Verification items for the finished model (mm, model axes). Face numbers are marked on the shaded views. A direction names the side the tool comes from. Give positions to 0.01 mm unless a question says otherwise; leave off trailing zeros. Write each loop counter-clockwise with the first axis right and the second up, starting at its lowest first coordinate (ties: lowest second). Pieces come first, ordered by that corner, then holes. Notation, with made-up numbers: (11.5, 13.5) - (56.5, 13.5) arc R9 ccw to (56.5, 26.5) - close; hole circle Ø10 at (-4, 39). An arc over 180 degrees is marked (long way). Put each result on its own line as item: value.
from build123d import *

# Parameters (mm, degrees)
SKETCH1_R           = 2
BOSS_EXTRUDE1_DEPTH = 1.6
SKETCH1_3_W         = 8.2
SKETCH1_3_H         = 8.2
SKETCH1_3_W_2       = 6.2
SKETCH1_3_H_2       = 6.2
BOSS_EXTRUDE2_DEPTH = 2
BOSS_EXTRUDE3_START = -0.5
SKETCH1_4_W         = 8.2
SKETCH1_4_H         = 8.2
SKETCH1_4_W_2       = 6.2
SKETCH1_4_H_2       = 6.2
SKETCH1_4_R         = 2
BOSS_EXTRUDE3_DEPTH = 0.5
SKETCH3_W           = 5.8
SKETCH3_H           = 5.8
BOSS_EXTRUDE4_DEPTH = 4.5
CHAMFER1_SIZE       = 0.5
CUT_EXTRUDE1_DEPTH  = 0.2


with BuildPart() as part:
    # Sketch1 → Boss-Extrude1 (new body)
    with BuildSketch(Plane(origin=(0, 0, 0), x_dir=(1, 0, 0), z_dir=(0, 1, 0))):
        with Locations(Location((0, 0, 0), (0, 0, 270))):
            Circle(SKETCH1_R)
    extrude(amount=BOSS_EXTRUDE1_DEPTH)



with BuildPart() as body_2:
    # Sketch1_3 → Boss-Extrude2 (new body)
    with BuildSketch(Plane(origin=(0, 0, 0), x_dir=(1, 0, 0), z_dir=(0, 1, 0))):
        Rectangle(SKETCH1_3_W, SKETCH1_3_H)
        Rectangle(SKETCH1_3_W_2, SKETCH1_3_H_2, mode=Mode.SUBTRACT)
    extrude(amount=BOSS_EXTRUDE2_DEPTH)


with BuildPart() as part_1:
    add(part.part)

    add(body_2.part)  # Boss-Extrude3 merges body 2
    # Sketch1_4 → Boss-Extrude3 (add)
    # profile 1 of 3: a face of its own
    with BuildSketch(Plane(origin=(0, 0, 0), x_dir=(1, 0, 0), z_dir=(0, 1, 0)).offset(BOSS_EXTRUDE3_START)):
        Rectangle(SKETCH1_4_W, SKETCH1_4_H)
        Rectangle(SKETCH1_4_W_2, SKETCH1_4_H_2, mode=Mode.SUBTRACT)
    # profile 2 of 3: a face of its own
    with BuildSketch(Plane(origin=(0, 0, 0), x_dir=(1, 0, 0), z_dir=(0, 1, 0)).offset(BOSS_EXTRUDE3_START)):
        Rectangle(SKETCH1_4_W_2, SKETCH1_4_H_2)
        with Locations(Location((0, 0, 0), (0, 0, 270))):
            Circle(SKETCH1_4_R, mode=Mode.SUBTRACT)
    # profile 3 of 3: a face of its own
    with BuildSketch(Plane(origin=(0, 0, 0), x_dir=(1, 0, 0), z_dir=(0, 1, 0)).offset(BOSS_EXTRUDE3_START)):
        with Locations(Location((0, 0, 0), (0, 0, 270))):
            Circle(SKETCH1_4_R)
    extrude(amount=BOSS_EXTRUDE3_DEPTH)

    # Sketch3 → Boss-Extrude4 (add)
    with BuildSketch(Plane.XZ.offset(0.5)):
        Rectangle(SKETCH3_W, SKETCH3_H)
    extrude(amount=BOSS_EXTRUDE4_DEPTH)

    # Chamfer1
    chamfer1_edges = [part_1.edges().sort_by_distance(p)[0] for p in [
        (2.9, -2.75, -2.9),
        (2.9, -2.75, 2.9),
        (-2.9, -2.75, 2.9),
        (-2.9, -2.75, -2.9),
        (-4.1, 0.75, -4.1),
        (4.1, 0.75, -4.1),
        (4.1, 0.75, 4.1),
        (-4.1, 0.75, 4.1),
    ]]
    chamfer(chamfer1_edges, length=CHAMFER1_SIZE)

    # Sketch4 → Cut-Extrude1 (cut)
    with BuildSketch(Plane.XZ.offset(5)):
        Polygon((0.178918545, 2.162051717), (1.79430316, -1.337948283), (1.452856846, -1.337948283), (0.935428962, -0.216153411), (-0.65120966, -0.216153411), (-1.183361102, -1.337948283), (-1.52620966, -1.337948283), (0.13404675, 2.162051717), align=None)
        Polygon((0.152977039, 1.479860211), (-0.480837064, 0.142820948), (0.769964218, 0.142820948), align=None, mode=Mode.SUBTRACT)
    extrude(amount=-CUT_EXTRUDE1_DEPTH, mode=Mode.SUBTRACT)


solid = part_1.part
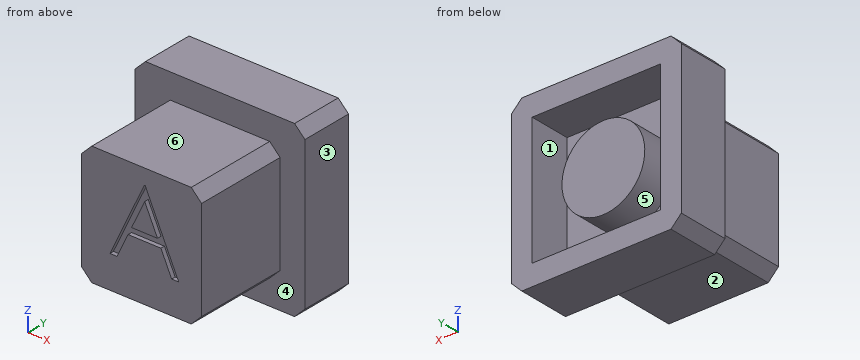
Q1. Scan lines: line 1 along X through (y, z) = (1.5, 0); line 2 along X through (y, z) = (1, -2.25). Record each from-to range of solid material in increasing order.
Answers follow:
line 1: x = -4.1 to -3.1, -2 to 2, 3.1 to 4.1
line 2: x = -4.1 to -3.1, 3.1 to 4.1
Q2. Release check for a two-part mould opening along X. For the marked faces 1, 2 and 3 record: released by +X, released by -X, zero draft, split by the parting line, or undercut.
Answers follow:
face 1: undercut
face 2: zero draft
face 3: released by +X
Q3. Section check B-B, the plane z = -2.75. Record the cut outline in (x, y).
Answers follow:
outline: (-4.1, -0.5) - (-2.55, -0.5) - (-2.55, -5) - (2.55, -5) - (2.55, -0.5) - (4.1, -0.5) - (4.1, 2) - (3.1, 2) - (3.1, 0) - (-3.1, 0) - (-3.1, 2) - (-4.1, 2) - close
Q4. Go/stop test with flat-tipped pins: pin 1 Ø2 at (x, z) = (-0.5, -0.5) entering from +Y; pin 2 Ø4 at (y, z) = (-3, 0.5) entering from +X; pin 3 Ø1.3 at (y, z) = (-2, 0.5) entering from -X. Record where each tip stops, or that it passes through.
Answers follow:
pin 1: stops at y = 1.6
pin 2: stops at x = 2.9
pin 3: stops at x = -2.9
Q5. Set-up check for the marked faces 4, 5 and 6: record each of +Z, -Z, +X, -X, +Y, -Y from which the full face is reachable in a straight line by a thin tool's end or side.
Answers follow:
face 4: -Y
face 5: +Y
face 6: +Z, +X, -X, -Y
Q6. Section check D-D, the plane y = -1.25. Record the cut outline in (x, z), plus the area to 3 significant figures.
Answers follow:
outline: (-2.9, -2.4) - (-2.4, -2.9) - (2.4, -2.9) - (2.9, -2.4) - (2.9, 2.4) - (2.4, 2.9) - (-2.4, 2.9) - (-2.9, 2.4) - close
area: 33.1 mm2
Q7. Section check A-A, the plane y = 0.5. Record the cut outline in (x, z).
Answers follow:
outline: (-4.1, -3.6) - (-3.6, -4.1) - (3.6, -4.1) - (4.1, -3.6) - (4.1, 3.6) - (3.6, 4.1) - (-3.6, 4.1) - (-4.1, 3.6) - close; circle Ø4 at (0, 0); hole (-3.1, -3.1) - (3.1, -3.1) - (3.1, 3.1) - (-3.1, 3.1) - close
Q8. Section check C-C, the plane x = 2.25. Record the cut outline in (y, z), plus the area to 3 significant figures.
Answers follow:
outline: (-5, -2.9) - (-0.5, -2.9) - (-0.5, -4.1) - (2, -4.1) - (2, -3.1) - (0, -3.1) - (0, 3.1) - (2, 3.1) - (2, 4.1) - (-0.5, 4.1) - (-0.5, 2.9) - (-5, 2.9) - close
area: 34.2 mm2
